The figure shows three views and two pictorial views of one solid part (mm, origin at its lowest corner). Answer the questions. A direction names the side the tool comes from. Round coordinates to 2 decimals unless told otherwise and drop trailing zeros. Order: outer loops, then holes, each group sorted by start corner. A loop starts at its lowest first (then second) coordinate and runs counter-clockwise, first axis right, second up. Notation, with made-up numbers: (77, 48) - (115, 48) arc R10 ccw to (115, 53) - close; hole circle Ø5 at (35, -17.5). An arc over 180 degrees is marked (long way). One line per item, written item: value. Start each with the question number.
1. Section A-A, the plane z = 1.5 is taken. Give the vertices of the cut face in (x, y), then the cut area to 3 significant figures.
2. Straight lines are drawn through the part: line 1 (Y direction, x = 9, z = 5); line 2 (X direction, y = 28, z = 19); line 3 (Z direction, x = 21, y = 3.5). For each, find the intervals that lie inside material, in ascending order.
3. For a pull along Y with two mould halves and no side action, classify the marked faces 1, 2 and 3 as released by +Y, released by -Y, zero draft, split by the parting line, or undercut.
4. Section B-B, the plane y = 52.5 is taken. Give the vertices of the cut face in (x, z).
5. Section C-C, the plane x = 8.5 is taken. Give the vertices of the cut face in (y, z), then the cut area to 3 significant figures.
6. A tool of negligible diameter and unlimited length cuts with its end or side. For the marked faces 4 and 5, from which of +Z, -Z, +X, -X, +Y, -Y can it reach the whole face along a straight path? Write none if from no direction.
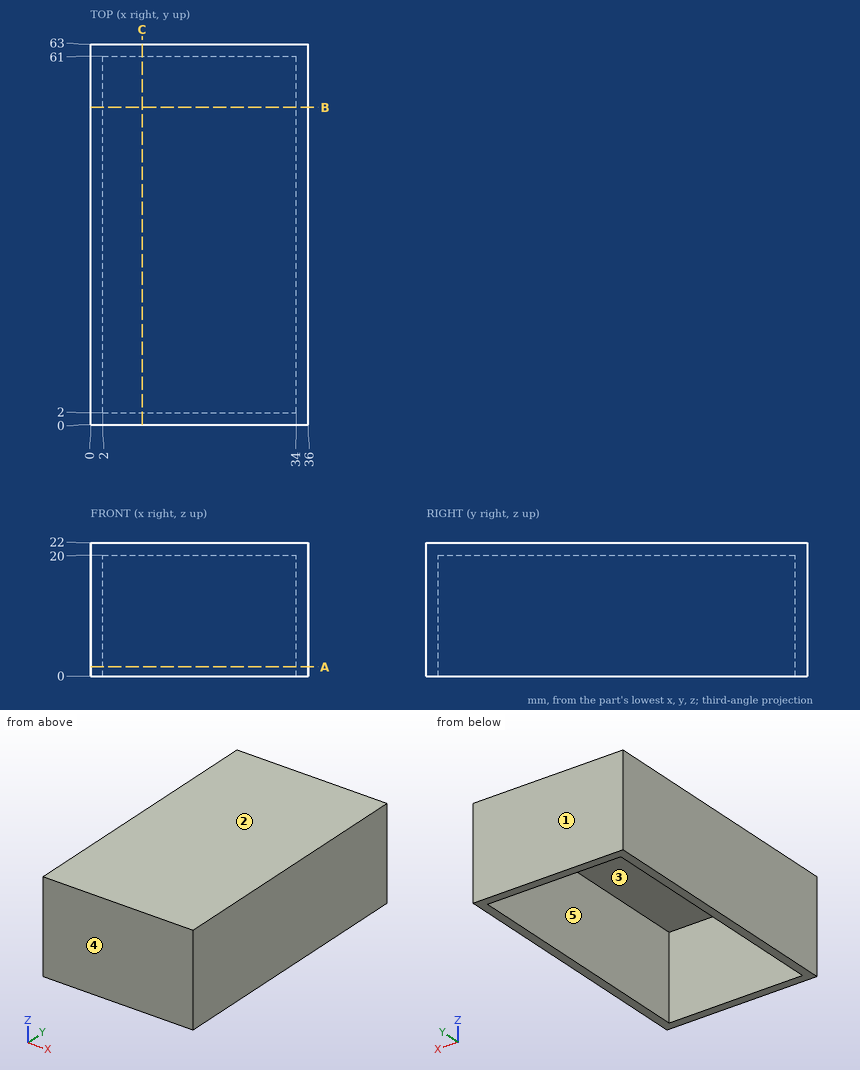
Answer list:
1. outline: (0, 0) - (36, 0) - (36, 63) - (0, 63) - close; hole (2, 2) - (34, 2) - (34, 61) - (2, 61) - close
1. area: 380 mm²
2. line 1: y = 0 to 2, 61 to 63
2. line 2: x = 0 to 2, 34 to 36
2. line 3: z = 20 to 22
3. face 1: released by +Y
3. face 2: zero draft
3. face 3: undercut
4. outline: (0, 0) - (2, 0) - (2, 20) - (34, 20) - (34, 0) - (36, 0) - (36, 22) - (0, 22) - close
5. outline: (0, 0) - (2, 0) - (2, 20) - (61, 20) - (61, 0) - (63, 0) - (63, 22) - (0, 22) - close
5. area: 206 mm²
6. face 4: +Z, -Z, +X, -X, -Y
6. face 5: -Z
